The figure shows three views and two pictorial views of one solid part (mm, origin at its lowest corner). Answer the questions. Coordinates: 2 decimals unless noted, no trailing zeros. Loops run counter-clockwise (first coordinate to the right, second up) from the corner with the lowest first, then second, coordinate; pieces in that order, holes last.
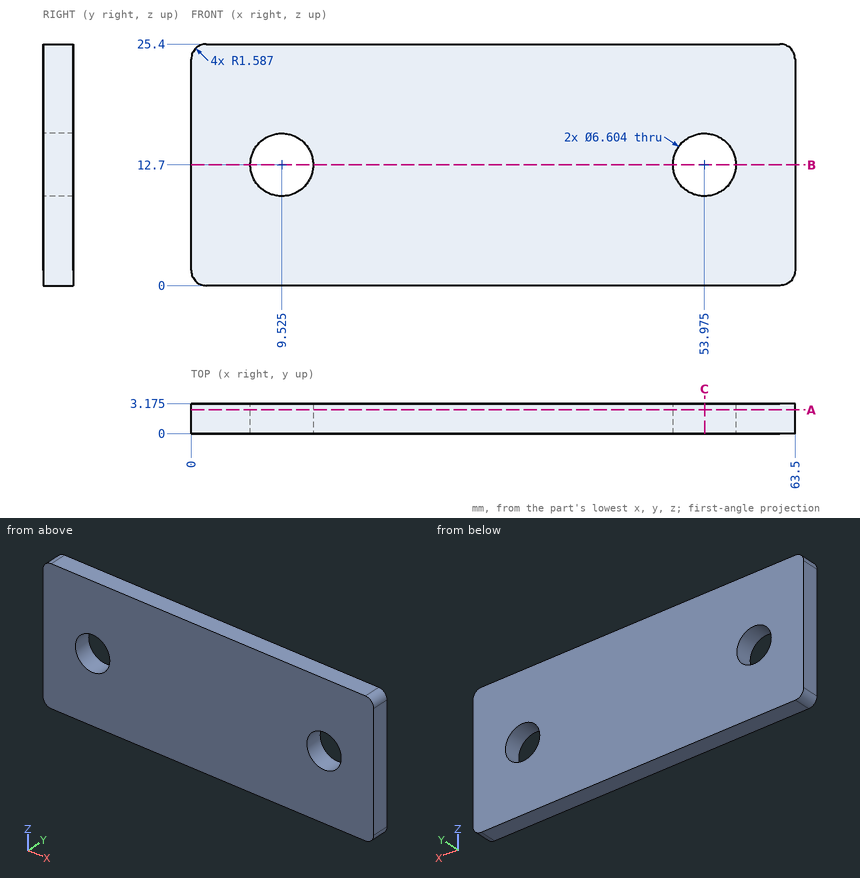
Q1. A flat-ended cylindrical pin translates along its axis: pin 1 Ø1 at (x, z) = (41.5, 13) entering from -Y. Find the tip coordinate at first contact, or state that the pin passes through.
Findings below:
pin 1: stops at y = 0
Q2. A cutting plane is placed at A-A (y = 2.5). Give the vertices of the cut face in (x, z) (1 decimal), then the cut area to 3 significant figures.
Findings below:
outline: (0, 1.6) arc R1.6 ccw to (1.6, 0) - (61.9, 0) arc R1.6 ccw to (63.5, 1.6) - (63.5, 23.8) arc R1.6 ccw to (61.9, 25.4) - (1.6, 25.4) arc R1.6 ccw to (0, 23.8) - close; hole circle Ø6.6 at (9.5, 12.7); hole circle Ø6.6 at (54, 12.7)
area: 1,540 mm2
Q3. A cutting plane is placed at B-B (z = 12.7). Give the vertices of the cut face in (x, y) (1 decimal).
Findings below:
outline: (0, 0) - (6.2, 0) - (6.2, 3.2) - (0, 3.2) - close; (12.8, 0) - (50.7, 0) - (50.7, 3.2) - (12.8, 3.2) - close; (57.3, 0) - (63.5, 0) - (63.5, 3.2) - (57.3, 3.2) - close
Q4. A cutting plane is placed at C-C (x = 54). Give the vertices of the cut face in (y, z) (1 decimal).
Findings below:
outline: (0, 0) - (3.2, 0) - (3.2, 9.4) - (0, 9.4) - close; (0, 16) - (3.2, 16) - (3.2, 25.4) - (0, 25.4) - close
Q5. Straight lines are drawn through the part: probe 1 along X at (y, z) = (0.3, 14); probe 2 along X at (y, z) = (2.9, 14.25); probe 3 along X at (y, z) = (0.85, 24). For each, find the intervals that lie inside material, in ascending order.
Findings below:
probe 1: x = 0 to 6.49, 12.56 to 50.94, 57.01 to 63.5
probe 2: x = 0 to 6.61, 12.44 to 51.06, 56.89 to 63.5
probe 3: x = 0.01 to 63.49
